```python
from build123d import *

# Parameters (mm, degrees)
TUBO_RETANGULAR_50_X_30_X_2_6_1_DEPTH = 535
ESBO_O2_R                             = 2.75
CORTE_EXTRUS_O1_DEPTH                 = 538.476743683


with BuildPart() as part:
    # Sketch1 → Tubo retangular 50 X 30 X 2.6(1) (new body)
    with BuildSketch(Plane.YZ):
        with BuildLine():
            Line((-9.5, -25), (9.5, -25))
            ThreePointArc((9.5, -25), (11.621320344, -24.121320344), (12.5, -22))
            Line((12.5, -22), (12.5, 22))
            ThreePointArc((12.5, 22), (11.621320344, 24.121320344), (9.5, 25))
            Line((9.5, 25), (-9.5, 25))
            ThreePointArc((-9.5, 25), (-11.621320344, 24.121320344), (-12.5, 22))
            Line((-12.5, 22), (-12.5, -22))
            ThreePointArc((-12.5, -22), (-11.621320344, -24.121320344), (-9.5, -25))
        make_face()
        with BuildLine():
            Line((-9.5, -22.4), (9.5, -22.4))
            ThreePointArc((9.5, -22.4), (9.782842712, -22.282842712), (9.9, -22))
            Line((9.9, -22), (9.9, 22))
            ThreePointArc((9.9, 22), (9.782842712, 22.282842712), (9.5, 22.4))
            Line((9.5, 22.4), (-9.5, 22.4))
            ThreePointArc((-9.5, 22.4), (-9.782842712, 22.282842712), (-9.9, 22))
            Line((-9.9, 22), (-9.9, -22))
            ThreePointArc((-9.9, -22), (-9.782842712, -22.282842712), (-9.5, -22.4))
        make_face(mode=Mode.SUBTRACT)
    extrude(amount=TUBO_RETANGULAR_50_X_30_X_2_6_1_DEPTH)

    # Esboço2 → Corte-extrusão1 (cut, through all)
    with BuildSketch(Plane(origin=(0, 0, -25), x_dir=(-1, 0, 0), z_dir=(0, 0, -1))):
        with Locations((-179.973841655, 0.2)):
            Circle(ESBO_O2_R)
        with Locations((-239.973841655, 0.2)):
            Circle(ESBO_O2_R)
        with Locations((-299.973841655, 0.2)):
            Circle(ESBO_O2_R)
    extrude(amount=-CORTE_EXTRUS_O1_DEPTH, mode=Mode.SUBTRACT)


solid = part.part
```
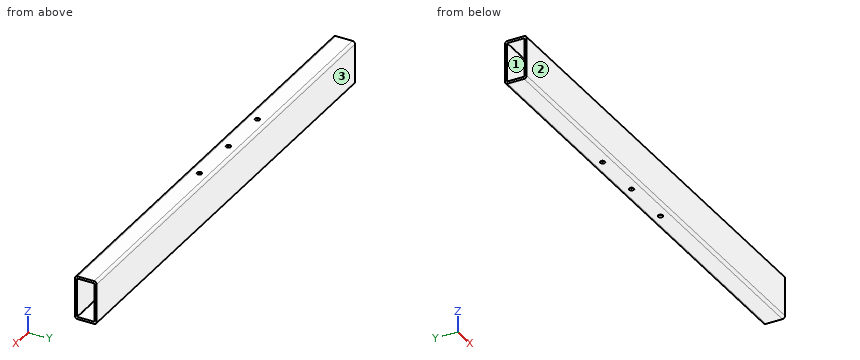
Design review of the part built by this model. Coordinates are the model's own, in mm. Face numbers are marked on the shaded views. Round coordinates to 2 decimals unless told otherwise and drop trailing zeros. Order: outer loops, then holes, each group sorted by start corner. A loop starts at its lowest first (then second) coordinate and runs counter-clockwise, first axis right, second up. Notation, with made-up numbers: (-40, 52.5) - (11, 52.5) arc R15 cw to (11, 73.5) - close; hole circle Ø7 at (51, 30). An arc over 180 degrees is marked (long way). Return JSON: item names as keys, results as strings.
Q1. Consider section A-A on z = -2.5. Write out the cut boundary in (x, y).
Computed values:
{"outline": "(0, -12.5) - (535, -12.5) - (535, -9.9) - (0, -9.9) - close; (0, 9.9) - (535, 9.9) - (535, 12.5) - (0, 12.5) - close"}
Q2. Consider section B-B on x = 201. Write out the cut boundary in (y, z), plus the area to 3 significant figures.
Computed values:
{"outline": "(-12.5, -22) arc R3 ccw to (-9.5, -25) - (9.5, -25) arc R3 ccw to (12.5, -22) - (12.5, 22) arc R3 ccw to (9.5, 25) - (-9.5, 25) arc R3 ccw to (-12.5, 22) - close; hole (-9.9, -22) arc R0.4 ccw to (-9.5, -22.4) - (9.5, -22.4) arc R0.4 ccw to (9.9, -22) - (9.9, 22) arc R0.4 ccw to (9.5, 22.4) - (-9.5, 22.4) arc R0.4 ccw to (-9.9, 22) - close", "area": "355 mm2"}
Q3. The part is to be moulded in two halves that separate along Y. For the marked faces 1, 2 and 3, say which applies: pulls with the +Y half, pulls with the -Y half, needs draft (parallel to the pull), parting line crosses it, or undercut.
Computed values:
{"face 1": "undercut", "face 2": "pulls with the -Y half", "face 3": "pulls with the +Y half"}
Q4. Wall thickness on L1, parallel to Z at x = 144.5, y = -4.25; L2, parallel to Y at x = 338, z = -16.5; L3, parallel to Z at x = 163.5, y = 10.25: over which ranges is each line inside the solid? List them lowest first. Write a range as [from, to].
Computed values:
{"L1": "z = [-25, -22.4], [22.4, 25]", "L2": "y = [-12.5, -9.9], [9.9, 12.5]", "L3": "z = [-24.9, 24.9]"}
